Model file for the job. Use its own axes, mm. A direction names the side the tool comes from. Coordinates: 2 decimals unless noted, no trailing zeros. Loops run counter-clockwise (first coordinate to the right, second up) from the corner with the lowest first, then second, coordinate; pieces in that order, holes last.
from build123d import *

# Parameters (mm, degrees)
SKETCH1_W           = 85
SKETCH1_H           = 46
BOSS_EXTRUDE1_DEPTH = 35
SKETCH3_R           = 12.5
CUT_EXTRUDE2_DEPTH  = 10
SKETCH4_R           = 3
CUT_EXTRUDE3_DEPTH  = 95.757585448
SKETCH2_W           = 80
SKETCH2_H           = 40
CUT_EXTRUDE4_DEPTH  = 60.667830529
SKETCH5_W           = 80
SKETCH5_H           = 40
BOSS_EXTRUDE2_DEPTH = 3
SKETCH6_R           = 19.25
SKETCH6_R_2         = 1.875
CUT_EXTRUDE6_DEPTH  = 1
BOSS_EXTRUDE3_START = 5
SKETCH7_R           = 1.875
BOSS_EXTRUDE3_DEPTH = 5


with BuildPart() as part:
    # Sketch1 → Boss-Extrude1 (new body)
    with BuildSketch(Plane(origin=(0, 0, 0), x_dir=(1, 0, 0), z_dir=(0, 1, 0))):
        Rectangle(SKETCH1_W, SKETCH1_H)
    extrude(amount=BOSS_EXTRUDE1_DEPTH)

    # Sketch3 → Cut-Extrude2 (cut)
    with BuildSketch(Plane(origin=(0, 0, -23), x_dir=(-1, 0, 0), z_dir=(0, 0, -1))):
        with Locations((0, 17.5)):
            Circle(SKETCH3_R)
    extrude(amount=-CUT_EXTRUDE2_DEPTH, mode=Mode.SUBTRACT)

    # Sketch4 → Cut-Extrude3 (cut, through all)
    with BuildSketch(Plane(origin=(42.5, 0, 0), x_dir=(0, 0, -1), z_dir=(1, 0, 0))):
        with Locations((0, 17.5)):
            Circle(SKETCH4_R)
    extrude(amount=-CUT_EXTRUDE3_DEPTH, mode=Mode.SUBTRACT)

    # Sketch2 → Cut-Extrude4 (cut, through all)
    with BuildSketch(Plane(origin=(0, 35, 0), x_dir=(1, 0, 0), z_dir=(0, 1, 0))):
        Rectangle(SKETCH2_W, SKETCH2_H)
    extrude(amount=-CUT_EXTRUDE4_DEPTH, mode=Mode.SUBTRACT)

    # Sketch5 → Boss-Extrude2 (add)
    with BuildSketch(Plane(origin=(0, 0, 0), x_dir=(1, 0, 0), z_dir=(0, 1, 0))):
        Rectangle(SKETCH5_W, SKETCH5_H)
    extrude(amount=BOSS_EXTRUDE2_DEPTH)

    # Sketch6 → Cut-Extrude6 (cut)
    with BuildSketch(Plane(origin=(0, 3, 0), x_dir=(1, 0, 0), z_dir=(0, 1, 0))):
        with Locations(Location((0, 0, 0), (0, 0, 270))):
            Circle(SKETCH6_R)
        with Locations(Location((0, 0, 0), (0, 0, 270))):
            Circle(SKETCH6_R_2, mode=Mode.SUBTRACT)
    extrude(amount=-CUT_EXTRUDE6_DEPTH, mode=Mode.SUBTRACT)

    # Sketch7 → Boss-Extrude3 (add)
    with BuildSketch(Plane(origin=(0, 3, 0), x_dir=(1, 0, 0), z_dir=(0, 1, 0)).offset(BOSS_EXTRUDE3_START)):
        with Locations(Location((0, 0, 0), (0, 0, 270))):
            Circle(SKETCH7_R)
    extrude(amount=-BOSS_EXTRUDE3_DEPTH)


solid = part.part
Q1. Flat gauge pins, fed straight in: P1, Ø20, axis at x = -9, z = -3, coming from the +Y side; P2, Ø4, axis at x = -25, z = 16.5, coming from the +Y side; P3, Ø1, axis at x = 5.5, z = 2, coming from the +Y side; P4, Ø5.5, axis at y = 17.5, z = 0, coming from the -X side. Where does each tip first touch, or does it go through?
Answers:
P1: stops at y = 8
P2: stops at y = 3
P3: stops at y = 2
P4: passes through
Q2. Slice it at C-C (x = 0). List the corners of the cut face in (y, z) (3 decimals), and give its area (3 significant figures).
Answers:
outline: (0, -23) - (5, -23) - (5, -20) - (3, -20) - (3, -19.25) - (2, -19.25) - (2, -1.875) - (8, -1.875) - (8, 1.875) - (2, 1.875) - (2, 19.25) - (3, 19.25) - (3, 20) - (35, 20) - (35, 23) - (0, 23) - close; (30, -23) - (35, -23) - (35, -20) - (30, -20) - close
area: 239 mm2
Q3. Slice it at B-B (y = 17.5). List the corners of the cut face in (x, z), and give its area (3 significant figures).
Answers:
outline: (-42.5, -23) - (-12.5, -23) - (-12.5, -20) - (-40, -20) - (-40, -3) - (-42.5, -3) - close; (-42.5, 3) - (-40, 3) - (-40, 20) - (40, 20) - (40, 3) - (42.5, 3) - (42.5, 23) - (-42.5, 23) - close; (12.5, -23) - (42.5, -23) - (42.5, -3) - (40, -3) - (40, -20) - (12.5, -20) - close
area: 605 mm2
Q4. Which spindle directions (+Z, -Z, +X, -X, +Y, -Y) get a long thin tool onto all of the face, cutting with end or side? Do faces 1 (the flat face through (0, 8, 0)), 2 (the cylindrical face through (-5.77, 6.41, -21.52)), 3 (the cylindrical face through (0.082, 5.042, -1.873)). Say none if no direction does.
Answers:
face 1: -Z, +Y
face 2: -Z
face 3: +Y
Q5. Slice it at A-A (z = 0). List the corners of the cut face in (x, y) (3 decimals), and give its area (3 significant figures).
Answers:
outline: (-42.5, 0) - (42.5, 0) - (42.5, 14.5) - (40, 14.5) - (40, 3) - (19.25, 3) - (19.25, 2) - (1.875, 2) - (1.875, 8) - (-1.875, 8) - (-1.875, 2) - (-19.25, 2) - (-19.25, 3) - (-40, 3) - (-40, 14.5) - (-42.5, 14.5) - close; (-42.5, 20.5) - (-40, 20.5) - (-40, 35) - (-42.5, 35) - close; (40, 20.5) - (42.5, 20.5) - (42.5, 35) - (40, 35) - close
area: 369 mm2
Q6. Mould opens along Y. For faces 4 (the flat face through (-1, 0, 0)), 5 (the flat face through (-18, 3, 9)), 6 (the flat face through (-10, 9, -23)), 7 (the cylindrical face through (41.27, 14.57, 0.65)) say: +Y half, -Y half, draft (parallel to the pull), parting line (faces both ways), or undercut.
Answers:
face 4: -Y half
face 5: +Y half
face 6: draft
face 7: undercut
Q7. Slice it at D-D (y = 25). List the corners of the cut face in (x, z), and give its area (3 significant figures).
Answers:
outline: (-42.5, -23) - (-10, -23) - (-10, -20) - (-40, -20) - (-40, 20) - (40, 20) - (40, -20) - (10, -20) - (10, -23) - (42.5, -23) - (42.5, 23) - (-42.5, 23) - close
area: 650 mm2
Q8. Drill centre lines: line 1 (X direction, y = 2.5, z = 0) (3 decimals); line 2 (Z direction, x = 33.5, y = 22); line 3 (Y direction, x = -41, z = 0). Where is each one in solid material? Low to high.
Answers:
line 1: x = -42.5 to -19.25, -1.875 to 1.875, 19.25 to 42.5
line 2: z = -23 to -20, 20 to 23
line 3: y = 0 to 14.5, 20.5 to 35
